Here's how the part is built. I have some questions about the finished solid (model axes, mm). A direction names the side the tool comes from. Coordinates: 2 decimals unless noted, no trailing zeros. Write each loop counter-clockwise with the first axis right and the second up, starting at its lowest first coordinate (ties: lowest second). Pieces come first, ordered by that corner, then holes. Notation, with made-up numbers: (22, -1) - (35, -1) arc R33 ccw to (35, 30) - close; hole circle Ø10 at (55, -35). An arc over 180 degrees is marked (long way). Answer in a Markdown table with one row per item. Add a question column.
Item 1: We'd pull the mould along Z, two halves only. Please class faces 4 (the face through (3.22, 74.71, 118.12)), 5 (the face through (3.131, 23.183, 62.05)), 6 (the face through (3.22, 151.62, 98.43)): +Z half, -Z half, draft (parallel to the pull), parting line (faces both ways), or undercut.
Item 2: I'm going to push flat-ended pins straight in: pin 1 (3 mm diameter, centred on x = 2.5, y = 105.5, fed in from -Z); pin 2 (2 mm diameter, centred on x = 1.5, y = 29, fed in from -Z); pin 3 (5.5 mm diameter, centred on y = 25.4, z = -16.12, fed in from -X); pin 4 (3 mm diameter, centred on x = 2, z = 60, fed in from +Y). Where does each tip first touch, or does it pass through?
Item 3: Imagine slicing it at D-D (y = 75.5). Please give me the cut outline in (x, z).
Item 4: If I drill on probe 1 along Z at (x, y) = (1, 49.5); probe 2 along Z at (x, y) = (3.5, 59); probe 3 along Y at (x, z) = (5, 71), over which ranges is the centre line in solid material (lowest first)? Write a range as from..to.
Item 5: Imagine slicing it at C-C (y = 12.7). Please give me the cut outline in (x, z).
Item 6: Imagine slicing it at A-A (z = 162.5). Please give me the cut outline in (x, y).
Item 7: Imagine slicing it at B-B (y = 50.8). Please give me the cut outline in (x, z).
Item 8: Which directions (+Z, -Z, +X, -X, +Y, -Y) give clear straight access to the entire face, cutting with the end or side of a thin tool? Please do faces 1 (the face through (3.22, 129.47, 163.52)), 2 (the face through (3, 140.459, 197)), 3 (the face through (3, 91.409, 191)).
from build123d import *

# Parameters (mm, degrees)
SKETCH1_W                 = 7.62
SKETCH1_H                 = 19.05
SKETCH1_H_2               = 18
BOSS_EXTRUDE1_DEPTH       = 6.35
FILLET1_R                 = 25.4
FILLET2_R                 = 12.7
M6_CLEARANCE_HOLE1_D      = 6.6
M3_CLEARANCE_HOLE1_D      = 3.4
M3_CLEARANCE_HOLE1_DEPTH  = 12.7
FILLET4_R                 = 15
M3X0_5_TAPPED_HOLE1_D     = 2.5
M3X0_5_TAPPED_HOLE1_DEPTH = 25.4
M3X0_5_TAPPED_HOLE1_TIP   = 0.751075774


with BuildPart() as part:
    # Sketch1 → Boss-Extrude1 (new body)
    with BuildSketch(Plane(origin=(0, 0, 0), x_dir=(0, 0, -1), z_dir=(1, 0, 0))):
        with BuildLine():
            Line((-28.329731999, 0), (124.070268001, 0))
            Line((124.070268001, 0), (-28.329731999, 104.775))
            Line((-28.329731999, 104.775), (-28.329731999, 83.211174444))
            Line((-28.329731999, 83.211174444), (-7.855401914, 69.135072511))
            ThreePointArc((-7.855401914, 69.135072511), (0.925492913, 37.798764283), (-28.329731999, 23.543935534))
            Line((-28.329731999, 23.543935534), (-28.329731999, 0))
        make_face()
        with BuildLine():
            Line((-28.329731999, 83.211174444), (-28.329731999, 104.775))
            Line((-28.329731999, 104.775), (-63.254731999, 128.7859375))
            Line((-63.254731999, 128.7859375), (-63.254731999, 105.242001966))
            ThreePointArc((-63.254731999, 105.242001966), (-58.93358663, 103.752256793), (-54.949397882, 101.512194739))
            Line((-54.949397882, 101.512194739), (-28.329731999, 83.211174444))
        make_face()
        with BuildLine():
            Line((-63.254731999, 105.242001966), (-63.254731999, 128.7859375))
            Line((-63.254731999, 128.7859375), (-98.179731999, 152.796875))
            Line((-98.179731999, 152.796875), (-98.179731999, 100.409375))
            Line((-98.179731999, 100.409375), (-90.269894858, 94.971361965))
            ThreePointArc((-90.269894858, 94.971361965), (-78.365507142, 104.323608978), (-63.254731999, 105.242001966))
        make_face()
        with BuildLine():
            Line((-98.179731999, 48.021875), (-63.254731999, 24.0109375))
            Line((-63.254731999, 24.0109375), (-63.254731999, 45.574763056))
            Line((-63.254731999, 45.574763056), (-83.729062085, 59.650864989))
            ThreePointArc((-83.729062085, 59.650864989), (-94.31459291, 75.956462655), (-90.269894858, 94.971361965))
            Line((-90.269894858, 94.971361965), (-98.179731999, 100.409375))
            Line((-98.179731999, 100.409375), (-98.179731999, 48.021875))
        make_face()
        with BuildLine():
            Line((-63.254731999, 24.0109375), (-28.329731999, 0))
            Line((-28.329731999, 0), (-28.329731999, 23.543935534))
            ThreePointArc((-28.329731999, 23.543935534), (-32.650877369, 25.033680707), (-36.635066117, 27.273742761))
            Line((-36.635066117, 27.273742761), (-63.254731999, 45.574763056))
            Line((-63.254731999, 45.574763056), (-63.254731999, 24.0109375))
        make_face()
        Polygon((-139.454731999, 48.021875), (-98.179731999, 48.021875), (-98.179731999, 100.409375), (-98.179731999, 152.796875), (-139.454731999, 152.796875), (-139.454731999, 133.746875), (-110.879731999, 133.746875), (-110.879731999, 67.071875), (-139.454731999, 67.071875), align=None)
        Polygon((-180.729731999, 48.021875), (-139.454731999, 48.021875), (-139.454731999, 67.071875), (-168.029731999, 67.071875), (-168.029731999, 133.746875), (-139.454731999, 133.746875), (-139.454731999, 152.796875), (-180.729731999, 152.796875), (-180.729731999, 121.409375), (-180.729731999, 109.409375), (-180.729731999, 100.409375), (-180.729731999, 91.409375), (-180.729731999, 79.409375), align=None)
        Polygon((-180.729731999, 121.409375), (-180.729731999, 152.796875), (-193.429731999, 152.796875), (-193.429731999, 140.459375), (-193.429731999, 121.409375), align=None)
        with Locations((-197.239731999, 130.934375)):
            Rectangle(SKETCH1_W, SKETCH1_H)
        Polygon((-193.429731999, 91.409375), (-180.729731999, 91.409375), (-180.729731999, 100.409375), (-180.729731999, 109.409375), (-193.429731999, 109.409375), align=None)
        with Locations((-197.239731999, 100.409375)):
            Rectangle(SKETCH1_W, SKETCH1_H_2)
        with Locations((-197.239731999, 69.884375)):
            Rectangle(SKETCH1_W, SKETCH1_H)
        Polygon((-193.429731999, 48.021875), (-180.729731999, 48.021875), (-180.729731999, 79.409375), (-193.429731999, 79.409375), (-193.429731999, 60.359375), align=None)
    extrude(amount=BOSS_EXTRUDE1_DEPTH)

    # Fillet1
    fillet1_edges = [part.edges().sort_by_distance(p)[0] for p in [
        (3.175, 67.071875, 110.879731999),
        (3.175, 133.746875, 110.879731999),
        (3.175, 152.796875, 98.179731999),
        (3.175, 48.021875, 98.179731999),
    ]]
    fillet(fillet1_edges, radius=FILLET1_R)

    # Fillet2
    fillet2_edges = [part.edges().sort_by_distance(p)[0] for p in [
        (3.175, 0, -124.070268001),
        (3.175, 0, 28.329731999),
    ]]
    fillet(fillet2_edges, radius=FILLET2_R)

    # M6 Clearance Hole1 (through all)
    with Locations(Plane(origin=(6.35, 0, 0), x_dir=(0, 0, -1), z_dir=(1, 0, 0))):
        with Locations((16.120268001, 25.4), (47.870268001, 25.4), (79.620268001, 12.7), (16.120268001, 50.8)):
            Hole(M6_CLEARANCE_HOLE1_D / 2)

    # M3 Clearance Hole1
    with Locations(Plane.XY.offset(180.729731999)):
        with Locations((3.175, 85.409375), (3.175, 115.409375)):
            Hole(M3_CLEARANCE_HOLE1_D / 2, depth=M3_CLEARANCE_HOLE1_DEPTH)

    # Fillet4
    fillet4_edges = [part.edges().sort_by_distance(p)[0] for p in [
        (3.175, 133.746875, 168.029731999),
        (3.175, 67.071875, 168.029731999),
    ]]
    fillet(fillet4_edges, radius=FILLET4_R)

    # M3x0.5 Tapped Hole1
    with Locations(Plane.XY.offset(201.049731999)):
        with Locations((3.175, 69.884375), (3.175, 130.934375), (3.175, 100.409375)):
            Hole(M3X0_5_TAPPED_HOLE1_D / 2, depth=M3X0_5_TAPPED_HOLE1_DEPTH)
            with Locations((0, 0, -(M3X0_5_TAPPED_HOLE1_DEPTH + M3X0_5_TAPPED_HOLE1_TIP / 2))):  # 118° drill point
                Cone(0, M3X0_5_TAPPED_HOLE1_D / 2, M3X0_5_TAPPED_HOLE1_TIP, mode=Mode.SUBTRACT)


solid = part.part
Here are the results:
| question | item | result |
|---|---|---|
| 1 | face 4 | undercut |
| 1 | face 5 | +Z half |
| 1 | face 6 | -Z half |
| 2 | pin 1 | stops at z = 27.2 |
| 2 | pin 2 | stops at z = -83.34 |
| 2 | pin 3 | passes through |
| 2 | pin 4 | stops at y = 127.58 |
| 3 | outline | (0, -14.25) - (6.35, -14.25) - (6.35, 17.11) - (0, 17.11) - close; (0, 94.23) - (6.35, 94.23) - (6.35, 117.38) - (0, 117.38) - close; (0, 166.51) - (6.35, 166.51) - (6.35, 201.05) - (0, 201.05) - close |
| 4 | probe 1 | z = -52.07..-19.15, -13.09..-3.12, 68.96..193.43 |
| 4 | probe 2 | z = -38.25..-0.75, 82.78..193.43 |
| 4 | probe 3 | y = 29.34..50.9, 105.93..134.11 |
| 5 | outline | (0, -95.88) - (6.35, -95.88) - (6.35, -82.92) - (0, -82.92) - close; (0, -76.32) - (6.35, -76.32) - (6.35, 46.8) - (0, 46.8) - close |
| 6 | outline | (0, 48.02) - (6.35, 48.02) - (6.35, 70.44) - (0, 70.44) - close; (0, 130.38) - (6.35, 130.38) - (6.35, 152.8) - (0, 152.8) - close |
| 7 | outline | (0, -50.18) - (6.35, -50.18) - (6.35, -19.42) - (0, -19.42) - close; (0, -12.82) - (6.35, -12.82) - (6.35, -3.02) - (0, -3.02) - close; (0, 70.86) - (6.35, 70.86) - (6.35, 193.43) - (0, 193.43) - close |
| 8 | face 1 | +X, -X |
| 8 | face 2 | +Z, +X, -X, +Y |
| 8 | face 3 | +Z, +X, -X |
